Read the model definition and answer for the solid it produces. Units are mm, in the model's axes. Give positions to 0.01 mm unless a question says otherwise; leave off trailing zeros. Order: outer loops, then holes, each group sorted by start corner. A loop starts at its lowest first (then second) coordinate and runs counter-clockwise, first axis right, second up.
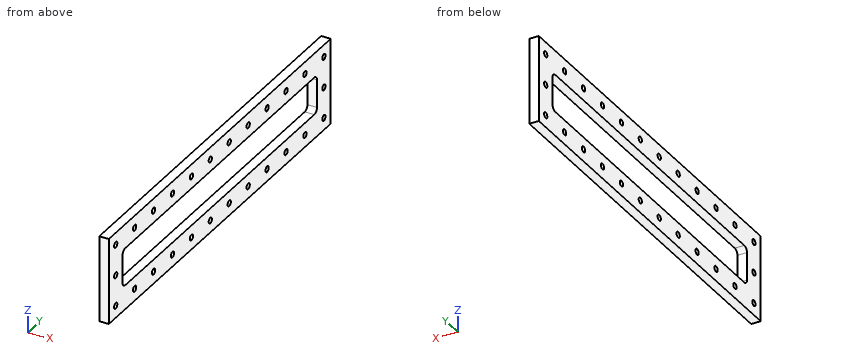
```python
from build123d import *

# Parameters (mm, degrees)
SKETCH1_W           = 90
SKETCH1_H           = 410.4
SKETCH1_R           = 3
BOSS_EXTRUDE1_DEPTH = 10


with BuildPart() as part:
    # Sketch1 → Boss-Extrude1 (new body)
    with BuildSketch(Plane(origin=(2615, 0, 0), x_dir=(0, 0, -1), z_dir=(1, 0, 0))):
        with Locations((-925, 999.8)):
            Rectangle(SKETCH1_W, SKETCH1_H)
        with Locations((-957.3, 807.3)):
            Circle(SKETCH1_R, mode=Mode.SUBTRACT)
        with Locations((-892.7, 807.3)):
            Circle(SKETCH1_R, mode=Mode.SUBTRACT)
        with Locations((-957.3, 842.3)):
            Circle(SKETCH1_R, mode=Mode.SUBTRACT)
        with Locations((-892.7, 842.3)):
            Circle(SKETCH1_R, mode=Mode.SUBTRACT)
        with Locations((-957.3, 877.3)):
            Circle(SKETCH1_R, mode=Mode.SUBTRACT)
        with Locations((-892.7, 877.3)):
            Circle(SKETCH1_R, mode=Mode.SUBTRACT)
        with Locations((-957.3, 912.3)):
            Circle(SKETCH1_R, mode=Mode.SUBTRACT)
        with Locations((-892.7, 912.3)):
            Circle(SKETCH1_R, mode=Mode.SUBTRACT)
        with Locations((-957.3, 947.3)):
            Circle(SKETCH1_R, mode=Mode.SUBTRACT)
        with Locations((-892.7, 947.3)):
            Circle(SKETCH1_R, mode=Mode.SUBTRACT)
        with Locations((-957.3, 982.3)):
            Circle(SKETCH1_R, mode=Mode.SUBTRACT)
        with Locations((-892.7, 982.3)):
            Circle(SKETCH1_R, mode=Mode.SUBTRACT)
        with Locations((-957.3, 1017.3)):
            Circle(SKETCH1_R, mode=Mode.SUBTRACT)
        with Locations((-892.7, 1017.3)):
            Circle(SKETCH1_R, mode=Mode.SUBTRACT)
        with Locations((-957.3, 1052.3)):
            Circle(SKETCH1_R, mode=Mode.SUBTRACT)
        with Locations((-892.7, 1052.3)):
            Circle(SKETCH1_R, mode=Mode.SUBTRACT)
        with Locations((-957.3, 1087.3)):
            Circle(SKETCH1_R, mode=Mode.SUBTRACT)
        with Locations((-892.7, 1087.3)):
            Circle(SKETCH1_R, mode=Mode.SUBTRACT)
        with Locations((-957.3, 1122.3)):
            Circle(SKETCH1_R, mode=Mode.SUBTRACT)
        with Locations((-892.7, 1122.3)):
            Circle(SKETCH1_R, mode=Mode.SUBTRACT)
        with Locations((-957.3, 1157.3)):
            Circle(SKETCH1_R, mode=Mode.SUBTRACT)
        with Locations((-892.7, 1157.3)):
            Circle(SKETCH1_R, mode=Mode.SUBTRACT)
        with Locations((-957.3, 1192.3)):
            Circle(SKETCH1_R, mode=Mode.SUBTRACT)
        with Locations((-892.7, 1192.3)):
            Circle(SKETCH1_R, mode=Mode.SUBTRACT)
        with Locations((-925, 807.3)):
            Circle(SKETCH1_R, mode=Mode.SUBTRACT)
        with Locations((-925, 1192.3)):
            Circle(SKETCH1_R, mode=Mode.SUBTRACT)
        with BuildLine():
            Line((-939.6, 1179.6), (-910.4, 1179.6))
            ThreePointArc((-910.4, 1179.6), (-906.864466094, 1178.135533906), (-905.4, 1174.6))
            Line((-905.4, 1174.6), (-905.4, 825))
            ThreePointArc((-905.4, 825), (-906.864466094, 821.464466094), (-910.4, 820))
            Line((-910.4, 820), (-939.6, 820))
            ThreePointArc((-939.6, 820), (-943.135533906, 821.464466094), (-944.6, 825))
            Line((-944.6, 825), (-944.6, 1174.6))
            ThreePointArc((-944.6, 1174.6), (-943.135533906, 1178.135533906), (-939.6, 1179.6))
        make_face(mode=Mode.SUBTRACT)
    extrude(amount=BOSS_EXTRUDE1_DEPTH)


solid = part.part
```
1) The part is cut by section B-B on y = 964. Determine the outline of the cut face in (x, z).
Final values:
outline: (2615, 880) - (2625, 880) - (2625, 905.4) - (2615, 905.4) - close; (2615, 944.6) - (2625, 944.6) - (2625, 970) - (2615, 970) - close
2) The part is cut by section A-A on z = 936. Determine the outline of the cut face in (x, y), and give its area (3 significant figures).
Final values:
outline: (2615, 794.6) - (2625, 794.6) - (2625, 820) - (2615, 820) - close; (2615, 1179.6) - (2625, 1179.6) - (2625, 1205) - (2615, 1205) - close
area: 508 mm2
3) Given pin 1 (9.5 mm diameter, centred on y = 842.3, z = 892.7, fed in from +X), flat-ended and moving along its own axis, determine where the tip first touches the part or whether it passes through.
Final values:
pin 1: stops at x = 2625
4) The part is cut by section C-C on x = 2619.75. Count the separate pieces of the cut face and the enclosed holes in it, and give its area (3 significant figures).
Final values:
separate pieces: 1
enclosed holes: 27
area: 22,100 mm2
5) Consider L1, parallel to Y at x = 2622.5, z = 925; L2, parallel to Z at x = 2623, y = 807.3; L3, parallel to Z at x = 2623.25, y = 1098. Determine where each line is inside the solid, lowest interval first.
Final values:
L1: y = 794.6 to 804.3, 810.3 to 820, 1179.6 to 1189.3, 1195.3 to 1205
L2: z = 880 to 889.7, 895.7 to 922, 928 to 954.3, 960.3 to 970
L3: z = 880 to 905.4, 944.6 to 970
